```python
from build123d import *

# Parameters (mm, degrees)
F0_R     = 11.2
F1_DEPTH = 7


with BuildPart() as f1:
    # F0 (on Top) → F1 (new body)
    with BuildSketch(Plane.XY):
        Polygon((11.919819, 6.817446), (5.110128, 34.602866), (-6.570164, 34.310859), (-11.86399, 6.914143), (-32.522025, -12.875932), (-26.428993, -22.845358), (-0.055828, -13.731589), (27.411896, -21.726934), (32.999157, -11.465501), align=None)
        Circle(F0_R, mode=Mode.SUBTRACT)
    extrude(amount=F1_DEPTH)


solid = f1.part
```
Geometry: final body of the model. Coordinates: model frame, mm. A direction names the side the tool comes from. Round coordinates to 2 decimals unless told otherwise and drop trailing zeros. Order: outer loops, then holes, each group sorted by start corner. A loop starts at its lowest first (then second) coordinate and runs counter-clockwise, first axis right, second up. Notation, with made-up numbers: (18.25, 13) -> (70.25, 13) arc R17 cw to (70.25, 25) -> close; hole circle Ø5 at (68.25, -21.5). An arc over 180 degrees is marked (long way). Write each question's results on one line, items separated by ' | '.
Q1. Pull-direction query (Y, two-part tool) for faces 1 (the face through (-22.048, -2.842, 3.451)), 2 (the face through (-11.19, 0.49, 3.45)), 3 (the face through (30.166, -16.668, 3.451)); classes: released by +Y, released by -Y, zero draft, split by the parting line, or undercut.
Response values:
face 1: released by +Y | face 2: undercut | face 3: released by -Y
Q2. Section query B-B (z = 1). Output: boundary loops of the cut face in (x, y).
Response values:
outline: (-32.52, -12.88) -> (-26.43, -22.85) -> (-0.06, -13.73) -> (27.41, -21.73) -> (33, -11.47) -> (11.92, 6.82) -> (5.11, 34.6) -> (-6.57, 34.31) -> (-11.86, 6.91) -> close; hole circle Ø22.4 at (0, 0)
Q3. Pin query (flat end, axial travel): pin 1 Ø4 at (x, z) = (8, 4) entering from -Y; pin 2 Ø2 at (y, z) = (9, 2) entering from +X; pin 3 Ø1.5 at (y, z) = (-12.5, 3.5) entering from +X. Return the tip coordinate at first contact, or that it passes through.
Response values:
pin 1: y = -16.66 | pin 2: x = 11.63 | pin 3: x = 32.84
Q4. Section query D-D (x = -16.5). Output: boundary loops of the cut face in (y, z).
Response values:
outline: (-19.41, 0) -> (2.47, 0) -> (2.47, 7) -> (-19.41, 7) -> close
Q5. Section query A-A (y = 4). Output: boundary loops of the cut face in (x, z).
Response values:
outline: (-14.91, 0) -> (-10.46, 0) -> (-10.46, 7) -> (-14.91, 7) -> close; (10.46, 0) -> (15.17, 0) -> (15.17, 7) -> (10.46, 7) -> close
Q6. Access query for faces 4 (the face through (22.607, -2.452, 3.451)), 5 (the face through (-13.427, -18.352, 3.451)). Directions: +Z, -Z, +X, -X, +Y, -Y. A direction counts if a zero-diameter tool reaches every point of the face in a straight line with its end or side. Return the directions, or none.
Response values:
face 4: +Z, -Z, +X, +Y | face 5: +Z, -Z, -Y
Q7. Ray query, line 1 along Y through (x, z) = (0, 4.25); line 2 along Y through (x, z) = (2, 3.5); line 3 along X through (y, z) = (0.5, 4.5). Return the intervals inside material, ascending.
Response values:
line 1: -13.75 to -11.2, 11.2 to 34.48 | line 2: -14.33 to -11.02, 11.02 to 34.53 | line 3: -18.56 to -11.19, 11.19 to 19.2
Q8. Section query C-C (y = -18). Output: boundary loops of the cut face in (x, z).
Response values:
outline: (-29.39, 0) -> (-12.41, 0) -> (-12.41, 7) -> (-29.39, 7) -> close; (14.61, 0) -> (29.44, 0) -> (29.44, 7) -> (14.61, 7) -> close
